Model file for the job. Use its own axes, mm. A direction names the side the tool comes from. Round coordinates to 2 decimals unless told otherwise and drop trailing zeros. Order: outer loops, then holes, each group sorted by start corner. A loop starts at its lowest first (then second) coordinate and runs counter-clockwise, first axis right, second up. Notation, with made-up numbers: M 12.5,-17.75 L 17.5,-17.75 A7 ccw 17.5,-10.75 Z; hole C 49,68.25 d5. An arc over 180 degrees is marked long. Return JSON: item names as keys, results as strings. Group by question number.
Item 1: Slice it at C-C on z = 12.7. Write the cut outline in (x, y) (3 decimals), then the cut area to 3 significant figures.
Item 2: Which spindle directions (+Z, -Z, +X, -X, +Y, -Y) get a long thin tool onto all of the face, cutting with end or side? Do faces 4 (the face through (-79.961, 3.131, -81.675)), 5 (the face through (50.756, 3, 0)), 6 (the face through (-83, 3, 3.175)), 7 (the face through (-3.175, 3, -58)), 8 (the face through (81.675, 3.131, -79.961)). Say none if no direction does.
Item 3: Slice it at A-A on y = 1.5. Write the cut outline in (x, z) (3 decimals).
Item 4: Pull direction Z, two halves, no side cores. Call faces 1 (the face through (0, 3, 0)), 2 (the face through (3.175, 3, -56)), 3 (the face through (83, 3, -3.175)): pulls with the +Z half, pulls with the -Z half, needs draft (parallel to the pull), parting line crosses it, or undercut.
Item 5: Probe line 1 along X through (y, z) = (4.5, -65) (3 decimals); line 2 along X through (y, z) = (0.5, -44.5) (3 decimals); line 3 along Z through (x, y) = (93, 4.25) (3 decimals). List the from-to ranges inside material, lowest first.
Item 6: Slice it at D-D on x = 0. Write the cut outline in (y, z), then the cut area to 3 significant figures.
Item 7: Pin check, flat tips, straight feed: pin 1 Ø3 at (x, y) = (79.5, 3) entering from +Z; pin 2 Ø1.9 at (x, y) = (-81.5, 4.5) entering from +Z; pin 3 Ø1.5 at (x, y) = (31.5, 1.5) entering from +Z. Stop position of each tip, or through.
Item 8: Slice it at B-B on x = -71.5. Write the cut outline in (y, z) (3 decimals), then the cut area to 3 significant figures.
from build123d import *

# Parameters (mm, degrees)
SKETCH1_R           = 114.3
BOSS_EXTRUDE1_DEPTH = 6.35
CUT_EXTRUDE2_DEPTH  = 162.769287876
CUT_EXTRUDE3_DEPTH  = 162.769287876
CUT_EXTRUDE5_DEPTH  = 162.738127462
SKETCH6_R           = 3.175
CUT_EXTRUDE6_DEPTH  = 162.738127462


with BuildPart() as part:
    # Sketch1 → Boss-Extrude1 (new body)
    with BuildSketch(Plane(origin=(0, 0, 0), x_dir=(1, 0, 0), z_dir=(0, 1, 0))):
        with Locations(Location((0, 0, 0), (0, 0, 270))):
            Circle(SKETCH1_R)
    extrude(amount=BOSS_EXTRUDE1_DEPTH)

    # Sketch3 → Cut-Extrude2 (cut, through all)
    with BuildSketch(Plane(origin=(0, 6.35, 0), x_dir=(1, 0, 0), z_dir=(0, 1, 0))):
        Polygon((114.255894268, 3.175), (120.605894268, 3.175), (120.605894268, -3.175), (114.255894268, -3.175), (50.755894268, -3.175), (50.755894268, 3.175), align=None)
    extrude(amount=-CUT_EXTRUDE2_DEPTH, mode=Mode.SUBTRACT)

    # Sketch4 → Cut-Extrude3 (cut, through all)
    with BuildSketch(Plane(origin=(0, 6.35, 0), x_dir=(1, 0, 0), z_dir=(0, 1, 0))):
        Polygon((-50.755894268, -3.175), (-114.255894268, -3.175), (-120.605894268, -3.175), (-120.605894268, 3.175), (-114.255894268, 3.175), (-50.755894268, 3.175), align=None)
    extrude(amount=-CUT_EXTRUDE3_DEPTH, mode=Mode.SUBTRACT)

    # Sketch5 → Cut-Extrude5 (cut, through all)
    with BuildSketch(Plane(origin=(0, 6.35, 0), x_dir=(1, 0, 0), z_dir=(0, 1, 0))):
        Polygon((-3.175, 0), (3.175, 0), (3.175, 114.255894268), (3.175, 116.129613815), (-3.175, 116.129613815), (-3.175, 114.255894268), align=None)
    extrude(amount=-CUT_EXTRUDE5_DEPTH, mode=Mode.SUBTRACT)

    # Sketch6 → Cut-Extrude6 (cut, through all)
    with BuildSketch(Plane(origin=(0, 6.35, 0), x_dir=(1, 0, 0), z_dir=(0, 1, 0))):
        with Locations(Location((-12.7, -12.7, 0), (0, 0, 270))):
            Circle(SKETCH6_R)
    extrude(amount=-CUT_EXTRUDE6_DEPTH, mode=Mode.SUBTRACT)


solid = part.part
Output values:
{
 "1": {"outline": "M -113.592,0 L -15.875,0 L -15.875,6.35 L -113.592,6.35 Z; M -9.525,0 L 113.592,0 L 113.592,6.35 L -9.525,6.35 Z", "area": "1,400 mm²"},
 "2": {"face 4": "-Z, -X, +Y, -Y", "face 5": "+X, +Y, -Y", "face 6": "-X, +Y, -Y", "face 7": "-Z, +Y, -Y", "face 8": "-Z, +X, +Y, -Y"},
 "3": {"outline": "M -114.256,-3.175 A114.3 ccw -3.175,-114.256 L -3.175,0 L 3.175,0 L 3.175,-114.256 A114.3 ccw 114.256,-3.175 L 50.756,-3.175 L 50.756,3.175 L 114.256,3.175 A114.3 ccw -114.256,3.175 L -50.756,3.175 L -50.756,-3.175 Z; hole C -12.7,12.7 d6.35"},
 "4": {"face 1": "pulls with the -Z half", "face 2": "needs draft", "face 3": "undercut"},
 "5": {"line 1": "-94.019 to -3.175, 3.175 to 94.019", "line 2": "-105.282 to -3.175, 3.175 to 105.282", "line 3": "-66.449 to -3.175, 3.175 to 66.449"},
 "6": {"outline": "M 0,0 L 6.35,0 L 6.35,114.3 L 0,114.3 Z", "area": "726 mm²"},
 "7": {"pin 1": "z = 83.55", "pin 2": "z = 81.09", "pin 3": "z = 110.09"},
 "8": {"outline": "M 0,-89.175 L 6.35,-89.175 L 6.35,-3.175 L 0,-3.175 Z; M 0,3.175 L 6.35,3.175 L 6.35,89.175 L 0,89.175 Z", "area": "1,090 mm²"}
}
